from build123d import *

# Parameters (mm, degrees)
SKETCH11_R              = 6
CUT_EXTRUDE4_DEPTH      = 28.5
F_1_2_20_TAPPED_HOLE1_D = 11.50874
SKETCH14_R              = 6.35
CUT_EXTRUDE5_DEPTH      = 22.3
SKETCH15_R              = 3.175
CUT_EXTRUDE6_DEPTH      = 4


with BuildPart() as part:
    # Sketch1 → Revolve1 (revolve)
    with BuildSketch(Plane(origin=(0, 0, 0), x_dir=(0, 0, -1), z_dir=(1, 0, 0))):
        with BuildLine():
            Line((0.5, 19), (38, 19))
            Line((38, 19), (38, 18))
            Line((38, 18), (34.1, 14.1))
            Line((34.1, 14.1), (18.3, 14.1))
            Line((18.3, 14.1), (16.9, 12.7))
            Line((16.9, 12.7), (-16.6, 12.7))
            Line((-16.6, 12.7), (-17.9, 14))
            Line((-17.9, 14), (-17.9, 20.7))
            ThreePointArc((-17.9, 20.7), (-18.192893219, 21.407106781), (-18.9, 21.7))
            Line((-18.9, 21.7), (-20.3, 21.7))
            Line((-20.3, 21.7), (-20.3, 23.3))
            ThreePointArc((-20.3, 23.3), (-20.885786438, 24.714213562), (-22.3, 25.3))
            Line((-22.3, 25.3), (-27.5, 25.3))
            Line((-27.5, 25.3), (-27.5, 27.9))
            Line((-27.5, 27.9), (-23.3, 27.9))
            ThreePointArc((-23.3, 27.9), (-21.885786438, 28.485786438), (-21.3, 29.9))
            Line((-21.3, 29.9), (-21.3, 30.4))
            Line((-21.3, 30.4), (-18.2, 30.4))
            ThreePointArc((-18.2, 30.4), (-16.785786438, 30.985786438), (-16.2, 32.4))
            Line((-16.2, 32.4), (-16.2, 60.4))
            Line((-16.2, 60.4), (-8, 60.4))
            Line((-8, 60.4), (-8, 39.3))
            ThreePointArc((-8, 39.3), (-7.853553391, 38.946446609), (-7.5, 38.8))
            Line((-7.5, 38.8), (-7.45, 38.8))
            Line((-7.45, 38.8), (-7.45, 37.7))
            ThreePointArc((-7.45, 37.7), (-6.864213562, 36.285786438), (-5.45, 35.7))
            Line((-5.45, 35.7), (-3.6, 35.7))
            Line((-3.6, 35.7), (-3.6, 28.85))
            Line((-3.6, 28.85), (0, 25.25))
            Line((0, 25.25), (0, 19.5))
            ThreePointArc((0, 19.5), (0.146446609, 19.146446609), (0.5, 19))
        make_face()
    revolve(axis=Axis((0, 0, 0), (0, 0, 1)))

    # Sketch11 → Cut-Extrude4 (cut, through all)
    with BuildSketch(Plane.XY):
        with Locations((0, 50)):
            Circle(SKETCH11_R)
        with Locations((50, 0)):
            Circle(SKETCH11_R)
        with Locations((0, -50)):
            Circle(SKETCH11_R)
        with Locations((-50, 0)):
            Circle(SKETCH11_R)
    extrude(amount=CUT_EXTRUDE4_DEPTH, mode=Mode.SUBTRACT)

    # Sketch7 → LatheCutPocket (revolve, cut)
    with BuildSketch(Plane(origin=(0, 0, 0), x_dir=(0, 0, -1), z_dir=(1, 0, 0))):
        Polygon((-19.9, 28), (-17.9, 26), (-17.9, 0), (-30.163250858, 0), (-30.163250858, 25.3), (-30.163250858, 28), (-30.163250858, 34.511397797), (-21.3, 34.511397797), (-21.3, 28), align=None)
    revolve(axis=Axis((0, 0, 0), (0, 0, 1)), mode=Mode.SUBTRACT)

    # 1/2-20 Tapped Hole1 (through all)
    with Locations(Plane.XY.offset(16.2)):
        with Locations((18.215731381, 43.976665748), (43.976665748, -18.215731381), (-18.215731381, -43.976665748), (-43.976665748, 18.215731381)):
            Hole(F_1_2_20_TAPPED_HOLE1_D / 2)

    # Sketch14 → Cut-Extrude5 (cut, through all)
    with BuildSketch(Plane.XY):
        with Locations((33.658282784, 33.658282784)):
            Circle(SKETCH14_R)
        with Locations((44.254149062, 18.330668733)):
            Circle(SKETCH14_R)
        with Locations((33.658282784, -33.658282784)):
            Circle(SKETCH14_R)
        with Locations((18.330668733, -44.254149062)):
            Circle(SKETCH14_R)
        with Locations((-33.658282784, -33.658282784)):
            Circle(SKETCH14_R)
        with Locations((-44.254149062, -18.330668733)):
            Circle(SKETCH14_R)
        with Locations((-33.658282784, 33.658282784)):
            Circle(SKETCH14_R)
        with Locations((-18.330668733, 44.254149062)):
            Circle(SKETCH14_R)
    extrude(amount=CUT_EXTRUDE5_DEPTH, mode=Mode.SUBTRACT)

    # Sketch15 → Cut-Extrude6 (cut)
    with BuildSketch(Plane.XY.offset(17.9)):
        with Locations((0, 15.075)):
            Circle(SKETCH15_R)
    extrude(amount=-CUT_EXTRUDE6_DEPTH, mode=Mode.SUBTRACT)


solid = part.part
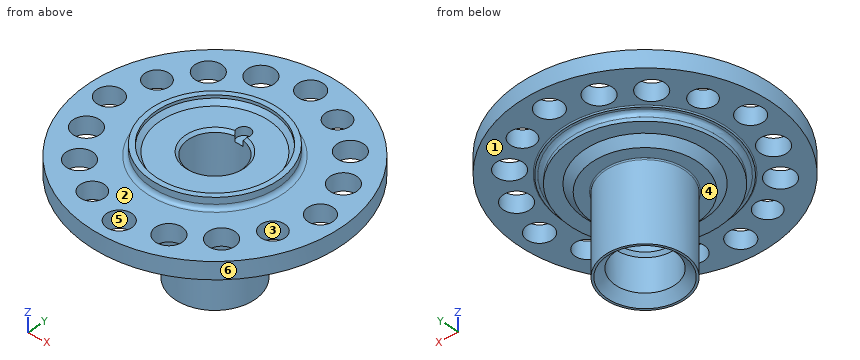
Input: part model. Units: mm. Frame: model coordinates. Face numbers are marked on the shaded views. A direction names the side the tool comes from. Give positions to 0.01 mm unless a question says otherwise; leave off trailing zeros. Loops run counter-clockwise (first coordinate to the right, second up) from the corner with the lowest first, then second, coordinate; pieces in that order, holes last. Notation, with made-up numbers: M 47.25,58.25 L 86.25,58.25 A24 ccw 86.25,75.25 Z; hole C 40.25,11 d8. An arc over 180 degrees is marked long. Use CSV: the item, a comma, the result in double quotes.
(1) Material intervals for L1, parallel to X at y = 0, z = 14; L2, parallel to Y at x = 0.5, z = 10; L3, parallel to X at y = 0, z = 20, sorted ascending. Write a range as [from, to].
Outcome:
L1,"x = [-60.4, -56], [-44, -12.7], [12.7, 44], [56, 60.4]"
L2,"y = [-60.4, -55.98], [-44.02, -12.69], [12.69, 44.02], [55.98, 60.4]"
L3,"x = [-30.4, -28], [28, 30.4]"
(2) Section B-B, the plane z = 11. Count the separate pieces of the cut face and the enclosed holes in it, plus the area to 3 significant figures.
Outcome:
separate pieces,"1"
enclosed holes,"17"
area,"9,070 mm²"
(3) Pull-direction query (Y, two-part tool) for the marked faces 4, 5 and 6; classes: pulls with the +Y half, pulls with the -Y half, needs draft (parallel to the pull), parting line crosses it, or undercut.
Outcome:
face 4,"needs draft"
face 5,"undercut"
face 6,"parting line crosses it"
(4) Section A-A, the plane z = -28. Return loops of the section in (x, y).
Outcome:
outline,"C 0,0 d38; hole C 0,0 d28.2"
(5) Pin query (flat end, axial travel): P1, Ø2, axis at y = -3, z = -5, coming from the -X side; P2, Ø13, axis at x = -43.98, y = 18.22, coming from the +Z side; P3, Ø3, axis at x = 27.5, y = -39, coming from the -Z side. Return the tip coordinate at first contact, or that it passes through.
Outcome:
P1,"stops at x = -18.89"
P2,"stops at z = 16.2"
P3,"stops at z = 8"
(6) Set-up query: the marked faces 1, 2 and 3. Return all of +Z, -Z, +X, -X, +Y, -Y with unobstructed straight access to the full face (end or side cutting, diameter ignored); none if empty.
Outcome:
face 1,"-Z"
face 2,"+Z"
face 3,"+Z, -Z"
